Model file for the job. Use its own axes, mm. Face numbers are marked on the shaded views. A direction names the side the tool comes from. Coordinates: 2 decimals unless noted, no trailing zeros. Write each loop counter-clockwise with the first axis right and the second up, starting at its lowest first coordinate (ties: lowest second). Pieces come first, ordered by that corner, then holes. Notation, with made-up numbers: M 2,84.5 L 9,84.5 A26 ccw 9,100.5 Z; hole C 88,-8 d1. An arc over 180 degrees is marked long. Answer in a Markdown table with one row per item. Add a question column.
```python
from build123d import *

# Parameters (mm, degrees)
F1_DEPTH  = 25.4
F2_R      = 6.35
F4_W      = 6.35
F4_H      = 88.9
F5_DEPTH  = 12.7
F6_W      = 6.35
F6_H      = 50.8
F5_FACE_W = 6.35
F5_FACE_H = 88.9
F8_W      = 88.9
F8_H      = 88.9
F9_DEPTH  = 6.35
F10_W     = 88.9
F10_H     = 88.9
F10_W_2   = 76.2
F10_H_2   = 76.2
F11_DEPTH = 3.175


with BuildPart() as f1:
    # F0 (on Top) → F1 (new body)
    with BuildSketch(Plane.XY):
        with BuildLine():
            ThreePointArc((0, 12.7), (12.7, 0), (0, -12.7))
            Line((0, -12.7), (-12.7, -12.7))
            Line((-12.7, -12.7), (-12.7, -25.4))
            Line((-12.7, -25.4), (38.1, -25.4))
            Line((38.1, -25.4), (38.1, 25.4))
            Line((38.1, 25.4), (-12.7, 25.4))
            Line((-12.7, 25.4), (-12.7, 12.7))
            Line((-12.7, 12.7), (0, 12.7))
        make_face()
    extrude(amount=F1_DEPTH)

    # F2
    f2_edges = [f1.edges().sort_by_distance(p)[0] for p in [
        (-12.7, -19.05, 25.4),
        (-12.7, 19.05, 25.4),
        (-12.7, -19.05, 0),
        (-12.7, 19.05, 0),
    ]]
    fillet(f2_edges, radius=F2_R)



with BuildPart() as f5:
    # F4 (on offset) → F5 (new body)
    with BuildSketch(Plane.XY.offset(-25.4)):
        with Locations((34.925, 0)):
            Rectangle(F4_W, F4_H)
    extrude(amount=F5_DEPTH)


with BuildPart() as f1_1:
    add(f1.part)

    add(f5.part)  # F7 merges F5
    # F6 (on face) → F7 section 0
    with BuildSketch(Plane.XY.offset(25.4)):
        with Locations((34.925, 0)):
            Rectangle(F6_W, F6_H)
    # F5_face (on face) → F7 section 1
    with BuildSketch(Plane(origin=(34.925, 0, -12.7), x_dir=(1, 0, 0), z_dir=(0, 0, 1))):
        Rectangle(F5_FACE_W, F5_FACE_H)
    loft()

    # F8 (on face) → F9 (join)
    with BuildSketch(Plane(origin=(0, 0, -25.4), x_dir=(1, 0, 0), z_dir=(0, 0, -1))):
        with Locations((82.55, 0)):
            Rectangle(F8_W, F8_H)
    extrude(amount=-F9_DEPTH)

    # F10 (on face) → F11 (join)
    with BuildSketch(Plane.XY.offset(-19.05)):
        with Locations((82.55, 0)):
            Rectangle(F10_W, F10_H)
        with Locations((82.55, 0)):
            Rectangle(F10_W_2, F10_H_2, mode=Mode.SUBTRACT)
    extrude(amount=F11_DEPTH)


solid = f1_1.part
```
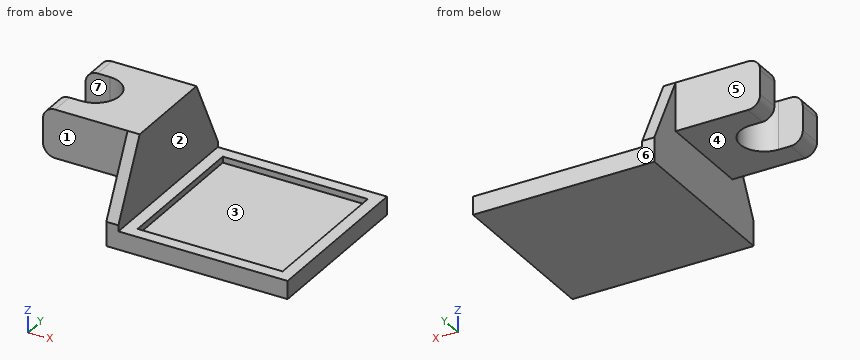
1) Flat gauge pins, fed straight in: pin 1 Ø8 at (y, z) = (-8.5, -14) entering from -X; pin 2 Ø1.5 at (x, y) = (17, -18.5) entering from -Z; pin 3 Ø10 at (x, z) = (-4.5, 16) entering from -Y; pin 4 Ø8 at (y, z) = (-28, 12) entering from -X. Where does each tip first touch, or does it go through?
2) Slice it at C-C (x = 115.5). Give the cut face in (y, z) (3 decimals), then the cut area to 3 significant figures.
3) Slice it at B-B (y = -21). Give the cut face in (x, z) (3 decimals).
4) Which spindle directions (+Z, -Z, +X, -X, +Y, -Y) get a long thin tool onto all of the face, cutting with end or side? Do the marked faces 4, 5, 6 and 7. Say none if no direction does.
5) Slice it at D-D (z = 9.5). Give the cut face in (x, y).
6) Slice it at A-A (z = -17.5). Give the cut face in (x, y), then the cut area to 3 significant figures.
7) Two-plate mould, pull along Y, no slides. Class the marked faces 1, 2 and 3: released by +Y, released by -Y, zero draft, split by the parting line, or undercut.
8) Drill centre lines: probe 1 along X at (y, z) = (32, -18.5); probe 2 along Z at (x, y) = (120.5, -10.5); probe 3 along Y at (x, z) = (24, 17). Where is each one in solid material? Low to high.
Ans:
| question | item | result |
|---|---|---|
| 1 | pin 1 | stops at x = 31.75 |
| 1 | pin 2 | stops at z = 0 |
| 1 | pin 3 | stops at y = -25.4 |
| 1 | pin 4 | stops at x = -12.7 |
| 2 | outline | M -44.45,-25.4 L 44.45,-25.4 L 44.45,-15.875 L 38.1,-15.875 L 38.1,-19.05 L -38.1,-19.05 L -38.1,-15.875 L -44.45,-15.875 Z |
| 2 | area | 605 mm2 |
| 3 | outline | M -12.7,6.35 A6.35 ccw -6.35,0 L 31.75,0 L 31.75,-25.4 L 127,-25.4 L 127,-15.875 L 120.65,-15.875 L 120.65,-19.05 L 44.45,-19.05 L 44.45,-15.875 L 38.1,-15.875 L 38.1,25.4 L -6.35,25.4 A6.35 ccw -12.7,19.05 Z |
| 4 | face 4 | -Z, -X, +Y, -Y |
| 4 | face 5 | +Z, -Z, -X, +Y |
| 4 | face 6 | +Z, -Z, +X, -X, +Y |
| 4 | face 7 | +Z, -Z, -X |
| 5 | outline | M -12.7,-25.4 L 31.75,-25.4 L 31.75,-33.35 L 38.1,-33.35 L 38.1,33.35 L 31.75,33.35 L 31.75,25.4 L -12.7,25.4 L -12.7,12.7 L 0,12.7 A12.7 cw 0,-12.7 L -12.7,-12.7 Z |
| 6 | outline | M 31.75,-44.45 L 127,-44.45 L 127,44.45 L 31.75,44.45 Z; hole M 44.45,-38.1 L 120.65,-38.1 L 120.65,38.1 L 44.45,38.1 Z |
| 6 | area | 2,660 mm2 |
| 7 | face 1 | released by -Y |
| 7 | face 2 | zero draft |
| 7 | face 3 | undercut |
| 8 | probe 1 | x = 31.75 to 44.45, 120.65 to 127 |
| 8 | probe 2 | z = -25.4 to -19.05 |
| 8 | probe 3 | y = -25.4 to 25.4 |
